The model under review builds one solid part; all positions refer to its coordinate system, in mm. A direction names the side the tool comes from. Give positions to 0.01 mm unless a question says otherwise; leave off trailing zeros. Order: outer loops, then holes, each group sorted by start corner. A loop starts at its lowest first (then second) coordinate and runs counter-clockwise, first axis right, second up. Notation, with made-up numbers: (-20, 57.25) - (28, 57.25) arc R26 cw to (28, 73.25) - close; hole circle Ø11 at (-23, 63.25). An arc over 180 degrees is marked (long way). Use CSV: the item, a comma, the result in double quotes.
```python
from build123d import *

# Parameters (mm, degrees)
SKETCH1_R           = 1.5
SKETCH1_W           = 5
SKETCH1_H           = 5
BOSS_EXTRUDE1_DEPTH = 5


with BuildPart() as part:
    # Sketch1 → Boss-Extrude1 (new body)
    with BuildSketch(Plane.XY):
        with BuildLine():
            Line((-95, 0), (95, 0))
            Line((95, 0), (95, 25.923215718))
            ThreePointArc((95, 25.923215718), (85.16818484, 41.770502039), (66.60299172, 40))
            ThreePointArc((66.60299172, 40), (39.84977522, 25.016488918), (10, 18))
            Line((10, 18), (10, 10))
            Line((10, 10), (-10, 10))
            Line((-10, 10), (-10, 18))
            ThreePointArc((-10, 18), (-39.84977522, 25.016488918), (-66.60299172, 40))
            ThreePointArc((-66.60299172, 40), (-85.16818484, 41.770502039), (-95, 25.923215718))
            Line((-95, 25.923215718), (-95, 0))
        make_face()
        with Locations((80.303300859, 14.696699141)):
            Circle(SKETCH1_R, mode=Mode.SUBTRACT)
        with Locations((69.696699141, 25.303300859)):
            Circle(SKETCH1_R, mode=Mode.SUBTRACT)
        with Locations(Location((-69.696699141, 25.303300859, 0), (0, 0, 180))):
            Circle(SKETCH1_R, mode=Mode.SUBTRACT)
        with Locations(Location((-80.303300859, 14.696699141, 0), (0, 0, 180))):
            Circle(SKETCH1_R, mode=Mode.SUBTRACT)
        with Locations((55, 7.5)):
            Circle(SKETCH1_R, mode=Mode.SUBTRACT)
        with Locations(Location((-55, 7.5, 0), (0, 0, 180))):
            Circle(SKETCH1_R, mode=Mode.SUBTRACT)
        Polygon((75, 12.928932188), (71.464466094, 9.393398282), (75, 5.857864376), (78.535533906, 9.393398282), align=None, mode=Mode.SUBTRACT)
        Polygon((82.071067812, 20), (85.606601718, 23.535533906), (89.142135624, 20), (85.606601718, 16.464466094), align=None, mode=Mode.SUBTRACT)
        Polygon((64.393398282, 23.535533906), (60.857864376, 20), (64.393398282, 16.464466094), (67.928932188, 20), align=None, mode=Mode.SUBTRACT)
        Polygon((71.464466094, 30.606601718), (75, 34.142135624), (78.535533906, 30.606601718), (75, 27.071067812), align=None, mode=Mode.SUBTRACT)
        Polygon((-64.393398282, 23.535533906), (-60.857864376, 20), (-64.393398282, 16.464466094), (-67.928932188, 20), align=None, mode=Mode.SUBTRACT)
        Polygon((-71.464466094, 30.606601718), (-75, 34.142135624), (-78.535533906, 30.606601718), (-75, 27.071067812), align=None, mode=Mode.SUBTRACT)
        Polygon((-75, 12.928932188), (-71.464466094, 9.393398282), (-75, 5.857864376), (-78.535533906, 9.393398282), align=None, mode=Mode.SUBTRACT)
        Polygon((-82.071067812, 20), (-85.606601718, 23.535533906), (-89.142135624, 20), (-85.606601718, 16.464466094), align=None, mode=Mode.SUBTRACT)
        with Locations((47.5, 7.5)):
            Rectangle(SKETCH1_W, SKETCH1_H, mode=Mode.SUBTRACT)
        with Locations((62.5, 7.5)):
            Rectangle(SKETCH1_W, SKETCH1_H, mode=Mode.SUBTRACT)
        with Locations((-47.5, 7.5)):
            Rectangle(SKETCH1_W, SKETCH1_H, mode=Mode.SUBTRACT)
        with Locations((-62.5, 7.5)):
            Rectangle(SKETCH1_W, SKETCH1_H, mode=Mode.SUBTRACT)
    extrude(amount=BOSS_EXTRUDE1_DEPTH)


solid = part.part
```
Item 1: Take a section at A-A, the plane y = 36. Give the boundary of the cut face in (x, z), and give its area (3 significant figures).
Results list:
outline,"(-91.85, 0) - (-60.99, 0) - (-60.99, 5) - (-91.85, 5) - close; (60.99, 0) - (91.85, 0) - (91.85, 5) - (60.99, 5) - close"
area,"309 mm2"
Item 2: Tool access review of faces 4 (the face through (95, 13, 2)), 5 (the face through (0, 10, 2)), 6 (the face through (-62.6, 18.26, 2.46)): name each direction out of +Z, -Z, +X, -X, +Y, -Y from which nothing blocks a thin tool from reaching the whole face with its end or side.
Results list:
face 4,"+Z, -Z, +X, +Y, -Y"
face 5,"+Z, -Z, +Y"
face 6,"+Z, -Z"
Item 3: Mouldability with a two-part tool opening along Y and no side actions: class faces 1 (the face through (62, 10, 2)), 2 (the face through (40.251, 25.173, 2.465)), 3 (the face through (-95, 13, 2)) as pulls with the +Y half, pulls with the -Y half, needs draft (parallel to the pull), parting line crosses it, or undercut.
Results list:
face 1,"undercut"
face 2,"pulls with the +Y half"
face 3,"needs draft"
Item 4: Take a section at C-C, the plane z = 3.9. State how many separate pieces and enclosed holes the cut face has, and give its area (3 significant figures).
Results list:
separate pieces,"1"
enclosed holes,"18"
area,"5,110 mm2"
Item 5: Clearance check with a flat-ended pin moving along its axis: pin 1 (2.5 mm diameter, centred on x = 48, z = 3.5, fed in from +Y). State where the tip first meets the part, or that it passes through.
Results list:
pin 1,"stops at y = 29.19"
Item 6: Take a section at B-B, the plane x = 5. Give the boundary of the cut face in (y, z).
Results list:
outline,"(0, 0) - (10, 0) - (10, 5) - (0, 5) - close"
Item 7: Wall thickness on L1, parallel to X at y = 17, z = 3.35; L2, parallel to Y at x = -73.5, z = 1.1; L3, parallel to X at y = 34, z = 3: over which ranges is each line inside the solid? List them lowest first.
Results list:
L1,"x = -95 to -86.14, -85.07 to -64.93, -63.86 to -10, 10 to 63.86, 64.93 to 85.07, 86.14 to 95"
L2,"y = 0 to 7.36, 11.43 to 28.57, 32.64 to 43.19"
L3,"x = -93.05 to -75.14, -74.86 to -57.87, 57.87 to 74.86, 75.14 to 93.05"
